Autodesk Inventor part; units mm, degrees
ref_plane "YZ Plane" through (0, 0, 0) normal (1, 0, 0) x (0, 1, 0)
ref_plane "XZ Plane" through (0, 0, 0) normal (0, 1, 0) x (-1, 0, 0)
ref_plane "XY Plane" through (0, 0, 0) normal (0, 0, 1) x (1, 0, 0)
sketch "Sketch1" plane through (0, 0, 0) normal (1, 0, 0) x (0, 1, 0)
  circle A0 centre (-37.5, 0) radius 5.5
  circle A1 centre (37.5, 0) radius 5.5
  line L0 (-50, 44) -> (50, 44)
  line L1 (50, 44) -> (50, -12.5)
  line L2 (50, -12.5) -> (-50, -12.5)
  line L3 (-50, -12.5) -> (-50, 44)
  point P0 (0, 0)
  dimension "d0" = 11
  dimension "d1" = 11
  dimension "d2" = 100
  dimension "d3" = 56.5
extrude "Extrusion1" add sketch "Sketch1" along normal blind 204
sketch "Sketch2" plane through (0, -50, -12.5) normal (0, -1, 0) x (1, 0, 0)
  line L0 (204, 0) -> (204, 56.5)
  line L1 (0, 0) -> (204, 0)
  line L2 (204, 0) -> (204, 56.5)
  line L3 (204, 56.5) -> (0, 56.5)
  line L4 (0, 56.5) -> (0, 0)
  line L5 (5.5, 0) -> (198.5, 0)
  line L6 (198.5, 0) -> (198.5, 46.5)
  line L7 (198.5, 46.5) -> (5.5, 46.5)
  line L8 (5.5, 46.5) -> (5.5, 0)
  point P0 (0, 12.5)
  point P1 (198.5, 0)
  dimension "d6" = 204
  dimension "d7" = 193
  dimension "d8" = 46.5
  dimension "d9" = 5.5
extrude "Extrusion2" cut sketch "Sketch2" against normal up to surface (100 mm away) contours L1 L8 L7 L6
sketch "Sketch3" plane through (204, 0, 0) normal (1, 0, 0) x (0, 0, -1)
  point P0 (0, 0)
fillet "Fillet1" radius 14 4 edges at (201.25, 50, -12.5) (201.25, -50, -12.5) (2.75, 50, -12.5) (2.75, -50, -12.5)
fillet "Fillet2" radius 2 2 edges at (198.5, 0, 34) (5.5, 0, 34)
fillet "Fillet3" radius 5 2 edges at (204, 0, 44) (0, 0, 44)
sketch "Sketch4" plane through (196.5, -50, 34) normal (0, 0, -1) x (-1, 0, 0)
  line L0 (0, 100) -> (189, 100)
  line L1 (58.5, 100) -> (118.5, 100)
  line L2 (118.5, 100) -> (118.5, 58)
  line L3 (118.5, 58) -> (58.5, 58)
  line L4 (58.5, 58) -> (58.5, 100)
  circle A0 centre (64.9, 80) radius 4
  circle A1 centre (114.9, 64) radius 4
  line L5 (-7.5, 14) -> (-7.5, 86)
  line L6 (94.5, 58) -> (94.5, 100)
  line L7 (196.5, 14) -> (196.5, 86)
  point P0 (196.5, 50)
  dimension "d15" = 60
  dimension "d16" = 42
  dimension "d17" = 8
  dimension "d19" = 6.4
  dimension "d20" = 8
  dimension "d22" = 6
  dimension "d24" = 36
  dimension "d25" = 102
  dimension "d26" = 204
  dimension "d34" = 16
  dimension "d36" = 50
extrude "Extrusion3" cut sketch "Sketch4" against normal blind 4 contours A1 L2 | L2 A1 | A0
sketch "Sketch5" plane through (131.6, 30, 38) normal (0, 0, -1) x (-1, 0, 0)
  circle A0 centre (0, 0) radius 4
  circle A1 centre (50, -16) radius 4
  circle A2 centre (0, 0) radius 2.125
  circle A3 centre (50, -16) radius 2.125
  point P0 (131.6, -30)
  dimension "d29" = 4.25
  dimension "d30" = 4.25
extrude "Extrusion4" cut sketch "Sketch5" against normal blind 6 contours A2 | A3
equation "\"d9\" = -0.5 * d7 + 0.5 * d6"
equation "\"d25\" = 0.5 * d26"
properties part number "LaserBeslag" material "PET Plastic"
Part model, mm, in its own coordinate system. A direction names the side the tool comes from. Coordinates: 2 decimals unless noted, no trailing zeros. Loops run counter-clockwise (first coordinate to the right, second up) from the corner with the lowest first, then second, coordinate; pieces in that order, holes last. Notation, with made-up numbers: (2, 31) - (27, 31) arc R8 cw to (27, 42) - close; hole circle Ø1 at (54, 61). An arc over 180 degrees is marked (long way). Write item = value, one per line. Start each with the question number.
Item 1: Cut at C-C, the plane y = -7.5. Give the cut face in (x, z), and give its area (3 significant figures).
Item 2: Cut at D-D, the plane y = 30. Give the cut face in (x, z) (3 decimals), and give its area (3 significant figures).
Item 3: Mould opens along X. For faces 4 (the cylindrical face through (201.3, 45.8, -8.5)), 5 (the cylindrical face through (1, 1, 42)), 6 (the cylindrical face through (133.723, 30.093, 40.958)) say: released by +X, released by -X, zero draft, split by the parting line, or undercut.
Item 4: Cut at A-A, the plane x = 131.6. Give the cut face in (y, z) (3 decimals), and give its area (4 significant figures).
Item 5: Wall check: L1, parallel to X at y = 33, z = 8; L2, parallel to X at y = 14, z = 36; L3, parallel to Y at x = 131.6, z = 41.2 (3 decimals). Give the ranges that are in metal, low to high. Write a range as from..to.
Item 6: 3-axis set-ups, long thin cutter, end or side, ignore diameter. For faces 1 (the flat face through (80, 12, 38)), 2 (the flat face through (198.5, -1, 9)), 3 (the flat face through (0, -1, 14)): which of +Z, -Z, +X, -X, +Y, -Y reach the whole face in a straight line?
Item 7: Cut at B-B, the plane z = 18. Give the cut face in (x, y), and give its area (3 significant figures).
Item 8: Flat gauge pins, fed straight in: pin 1 Ø10.5 at (x, y) = (81.6, 14) entering from -Z; pin 2 Ø14.5 at (y, z) = (37.5, 0) entering from +X; pin 3 Ø5 at (x, y) = (81.6, 14) entering from -Z; pin 4 Ø9 at (y, z) = (-37.5, 0) entering from +X. Where does each tip first touch, or does it go through?
The answers:
q1.outline = (0, -12.5) - (5.5, -12.5) - (5.5, 32) arc R2 cw to (7.5, 34) - (196.5, 34) arc R2 cw to (198.5, 32) - (198.5, -12.5) - (204, -12.5) - (204, 39) arc R5 ccw to (199, 44) - (5, 44) arc R5 ccw to (0, 39) - close
q1.area = 2,540 mm2
q2.outline = (0, -12.5) - (5.5, -12.5) - (5.5, 32) arc R2 cw to (7.5, 34) - (127.6, 34) - (127.6, 38) - (129.475, 38) - (129.475, 44) - (5, 44) arc R5 ccw to (0, 39) - close; (133.725, 38) - (135.6, 38) - (135.6, 34) - (196.5, 34) arc R2 cw to (198.5, 32) - (198.5, -12.5) - (204, -12.5) - (204, 39) arc R5 ccw to (199, 44) - (133.725, 44) - close
q2.area = 2,480 mm2
q3.face_4 = zero draft
q3.face_5 = released by -X
q3.face_6 = undercut
q4.outline = (-50, 34) - (26, 34) - (26, 38) - (27.875, 38) - (27.875, 44) - (-50, 44) - close; (32.125, 38) - (34, 38) - (34, 34) - (50, 34) - (50, 44) - (32.125, 44) - close
q4.area = 942.5 mm2
q5.L1 = 0..5.5, 198.5..204
q5.L2 = 0..77.6, 85.6..204
q5.L3 = -50..27.875, 32.125..50
q6.face_1 = -Z
q6.face_2 = -Z, +Y, -Y
q6.face_3 = +Z, -Z, -X, +Y, -Y
q7.outline = (0, -50) - (5.5, -50) - (5.5, 50) - (0, 50) - close; (198.5, -50) - (204, -50) - (204, 50) - (198.5, 50) - close
q7.area = 1,100 mm2
q8.pin_1 = 34
q8.pin_2 = 204
q8.pin_3 = 38
q8.pin_4 = through
